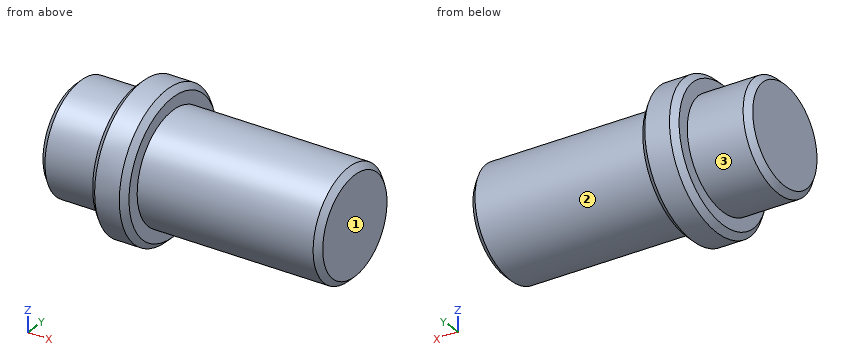
```python
from build123d import *

# Parameters (mm, degrees)
SKETCH1_R           = 2.38125
BOSS_EXTRUDE1_DEPTH = 12.2174
SKETCH2_R           = 3.175
BOSS_EXTRUDE2_DEPTH = 1.5875
CHAMFER1_SIZE       = 0.254


with BuildPart() as part:
    # Sketch1 → Boss-Extrude1 (new body)
    with BuildSketch(Plane(origin=(0, 0, 0), x_dir=(0, 0, -1), z_dir=(1, 0, 0))):
        Circle(SKETCH1_R)
    extrude(amount=BOSS_EXTRUDE1_DEPTH)

    # Sketch2 → Boss-Extrude2 (add)
    with BuildSketch(Plane.ZY.offset(-2.6924)):
        Circle(SKETCH2_R)
    extrude(amount=-BOSS_EXTRUDE2_DEPTH)

    # Chamfer1
    chamfer1_edges = [part.edges().sort_by_distance(p)[0] for p in [
        (0, 0, 2.38125),
        (12.2174, 0, 2.38125),
        (2.6924, 0, -3.175),
        (4.2799, 0, -3.175),
    ]]
    chamfer(chamfer1_edges, length=CHAMFER1_SIZE)


solid = part.part
```
Build history of the part. All positions in model axes, mm. Face numbers are marked on the shaded views. A direction names the side the tool comes from. Round coordinates to 2 decimals unless told otherwise and drop trailing zeros. Order: outer loops, then holes, each group sorted by start corner. A loop starts at its lowest first (then second) coordinate and runs counter-clockwise, first axis right, second up. Notation, with made-up numbers: (78.25, 89.25) -> (97.25, 89.25) arc R34 cw to (97.25, 124.25) -> close; hole circle Ø10 at (82, 71). An arc over 180 degrees is marked (long way). Answer in a Markdown table with one row per item.
1) Which spindle directions (+Z, -Z, +X, -X, +Y, -Y) get a long thin tool onto all of the face, cutting with end or side? Do the marked faces 1, 2 and 3. Say none if no direction does.
Values:
| item | result |
|---|---|
| face 1 | +Z, -Z, +X, +Y, -Y |
| face 2 | +X |
| face 3 | -X |
2) Band-saw the part on C-C on x = 9.5. Give the cut face in (y, z), and give its area (3 significant figures).
Values:
| item | result |
|---|---|
| outline | circle Ø4.76 at (0, 0) |
| area | 17.8 mm2 |
3) Wall check: L1, parallel to Z at x = 10, y = 0; L2, parallel to X at y = 0.25, z = 2.5; L3, parallel to Y at x = 4.5, z = 1.5. Give the ranges that are in metal, low to high.
Values:
| item | result |
|---|---|
| L1 | -2.38 to 2.38 |
| L2 | 2.69 to 4.28 |
| L3 | -1.85 to 1.85 |
4) Band-saw the part on A-A on y = 0. Give the cut face in (x, z) (3 decimals).
Values:
| item | result |
|---|---|
| outline | (0, -2.127) -> (0.254, -2.381) -> (2.692, -2.381) -> (2.692, -2.921) -> (2.946, -3.175) -> (4.026, -3.175) -> (4.28, -2.921) -> (4.28, -2.381) -> (11.963, -2.381) -> (12.217, -2.127) -> (12.217, 2.127) -> (11.963, 2.381) -> (4.28, 2.381) -> (4.28, 2.921) -> (4.026, 3.175) -> (2.946, 3.175) -> (2.692, 2.921) -> (2.692, 2.381) -> (0.254, 2.381) -> (0, 2.127) -> close |
5) Pin check, flat tip, straight feed: P1, Ø1, axis at x = 2.5, z = -2, coming from the +Y side. Stop position of the tip, or through.
Values:
| item | result |
|---|---|
| P1 | y = 2.63 |
